The drawing under review shows one solid part. Ordinate dimensions are in mm from its lowest x, y, z. A direction names the side the tool comes from. Coordinates: 2 decimals unless noted, no trailing zeros. Order: outer loops, then holes, each group sorted by start corner. A loop starts at its lowest first (then second) coordinate and runs counter-clockwise, first axis right, second up.
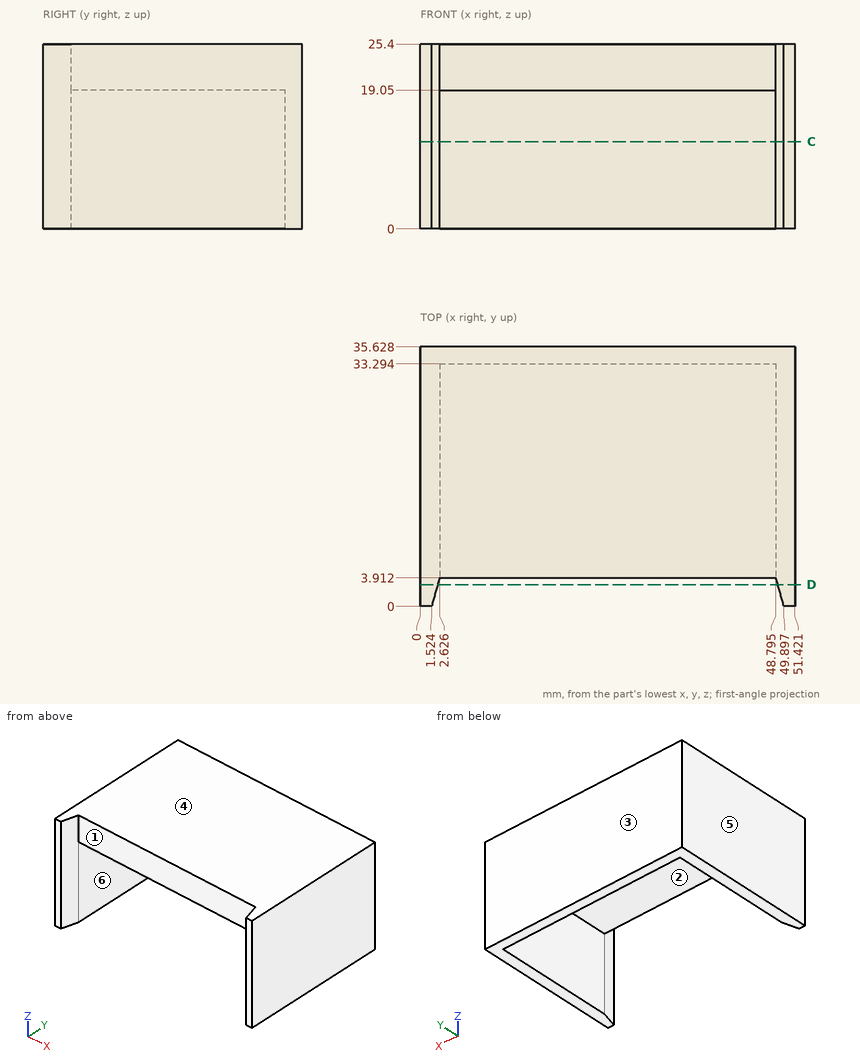
(1) Consider section D-D (y = 3). Give the boundary of the cut face in (x, z), then the cut area to 3 significant figures.
(2) The part is to be moulded in two halves that separate along X. For the marked faces 4, 5 and 6, say which applies: +X half, -X half, draft (parallel to the pull), parting line (faces both ways), or undercut.
(3) Tool access review of the marked faces 1, 2 and 3: name each direction out of +Z, -Z, +X, -X, +Y, -Y from which nothing blocks a thin tool from reaching the whole face with its end or side.
(4) Wall thickness on line 1 (X direction, y = 20, z = 11.25) (1 decimal); line 2 (Y direction, x = 28.5, z = 12.25) (1 decimal); line 3 (Z direction, x = 7, y = 5): over which ranges is each line inside the solid? List them lowest first.
(5) Consider section C-C (z = 12). Give the boundary of the cut face in (x, y) (1 decimal).
(6) Insertion check: pin 1 Ø9 at (x, y) = (16.5, 22.5) entering from -Z; pin 2 Ø9.5 at (x, z) = (37, 7) entering from -Y; pin 3 Ø3 at (x, z) = (35.5, 22.5) entering from -Y. Each pin has a flat end and moves straight along its axis. Give the tip position at first contact, or say it passes through.
Findings:
1. outline: (0, 0) - (2.37, 0) - (2.37, 25.4) - (0, 25.4) - close; (49.05, 0) - (51.42, 0) - (51.42, 25.4) - (49.05, 25.4) - close
1. area: 120 mm2
2. face 4: draft
2. face 5: -X half
2. face 6: undercut
3. face 1: +Z, -Z, -Y
3. face 2: -Z, -Y
3. face 3: +Z, -Z, +X, -X, +Y
4. line 1: x = 0 to 2.6, 48.8 to 51.4
4. line 2: y = 33.3 to 35.6
4. line 3: z = 19.05 to 25.4
5. outline: (0, 0) - (1.5, 0) - (2.6, 3.9) - (2.6, 33.3) - (48.8, 33.3) - (48.8, 3.9) - (49.9, 0) - (51.4, 0) - (51.4, 35.6) - (0, 35.6) - close
6. pin 1: stops at z = 19.05
6. pin 2: stops at y = 33.29
6. pin 3: stops at y = 3.91
